Work out the finished part from the listing and answer in its coordinate system (mm). Coordinates: 2 decimals unless noted, no trailing zeros. Order: outer loops, then holes, each group sorted by start corner. A loop starts at its lowest first (then second) coordinate and runs counter-clockwise, first axis right, second up. Notation, with made-up numbers: (85, 77.5) -> (135, 77.5) arc R23 cw to (135, 104.5) -> close; hole circle Ø4 at (-30.5, 4.25). An arc over 180 degrees is marked (long way). Use one line per item in the form item = value.
from build123d import *

# Parameters (mm, degrees)
SKETCH_W     = 43.2
SKETCH_H     = 10.2
PAD_DEPTH    = 25.4
SKETCH001_R  = 0.55
PAD001_DEPTH = 5.97
SKETCH002_R  = 1.5
POCKET_DEPTH = 25.401


with BuildPart() as part:
    # Sketch → Pad (new body)
    with BuildSketch(Plane.XY):
        Rectangle(SKETCH_W, SKETCH_H)
    extrude(amount=PAD_DEPTH)

    # Sketch001 (on Face5 of Pad) → Pad001 (join)
    with BuildSketch(Plane(origin=(0, 0, 0), x_dir=(1, 0, 0), z_dir=(0, 0, -1))):
        with Locations((14, 2.6)):
            Circle(SKETCH001_R)
        with Locations((3.8, 2.6)):
            Circle(SKETCH001_R)
        with Locations((-8.9, 2.6)):
            Circle(SKETCH001_R)
        with Locations((-14, 2.6)):
            Circle(SKETCH001_R)
        with Locations((-19, 2.6)):
            Circle(SKETCH001_R)
    extrude(amount=PAD001_DEPTH)

    # Sketch002 (on Face4 of Pad001) → Pocket (cut, through all)
    with BuildSketch(Plane(origin=(0, 0, 0), x_dir=(1, 0, 0), z_dir=(0, 0, -1))):
        with Locations((-3.8, -2.5)):
            Circle(SKETCH002_R)
    extrude(amount=-POCKET_DEPTH, mode=Mode.SUBTRACT)


solid = part.part
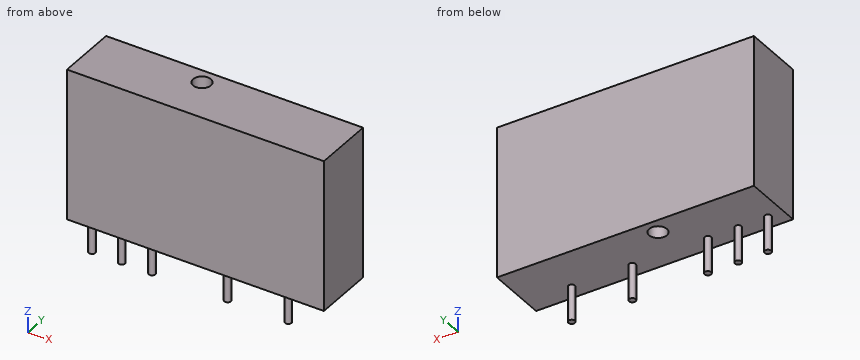
(1) Section B-B on y = 2.5 is taken. Write down the section's boundary in (x, z), plus the area to 3 significant figures.
Data:
outline = (-21.6, 0) -> (-5.3, 0) -> (-5.3, 25.4) -> (-21.6, 25.4) -> close; (-2.3, 0) -> (21.6, 0) -> (21.6, 25.4) -> (-2.3, 25.4) -> close
area = 1,020 mm²
(2) Straight lines are drawn through the part: line 1 along Y through (x, z) = (-3.8, 19.75); line 2 along X through (y, z) = (2.5, 17); line 3 along Z through (x, y) = (0, 0). For each, find the intervals that lie inside material, in ascending order.
Data:
line_1 = -5.1 to 1, 4 to 5.1
line_2 = -21.6 to -5.3, -2.3 to 21.6
line_3 = 0 to 25.4
(3) Section A-A on x = -3.8 is taken. Write down the section's boundary in (y, z).
Data:
outline = (-5.1, 0) -> (1, 0) -> (1, 25.4) -> (-5.1, 25.4) -> close; (4, 0) -> (5.1, 0) -> (5.1, 25.4) -> (4, 25.4) -> close
(4) Section D-D on y = -2.6 is taken. Write down the section's boundary in (x, z), plus the area to 3 significant figures.
Data:
outline = (-21.6, 0) -> (-19.55, 0) -> (-19.55, -5.97) -> (-18.45, -5.97) -> (-18.45, 0) -> (-14.55, 0) -> (-14.55, -5.97) -> (-13.45, -5.97) -> (-13.45, 0) -> (-9.45, 0) -> (-9.45, -5.97) -> (-8.35, -5.97) -> (-8.35, 0) -> (3.25, 0) -> (3.25, -5.97) -> (4.35, -5.97) -> (4.35, 0) -> (13.45, 0) -> (13.45, -5.97) -> (14.55, -5.97) -> (14.55, 0) -> (21.6, 0) -> (21.6, 25.4) -> (-21.6, 25.4) -> close
area = 1,130 mm²
(5) Section C-C on z = 15 is taken. Write down the section's boundary in (x, y).
Data:
outline = (-21.6, -5.1) -> (21.6, -5.1) -> (21.6, 5.1) -> (-21.6, 5.1) -> close; hole circle Ø3 at (-3.8, 2.5)
(6) This flat-tipped pin is pushed along its axis until it touches: P1, Ø5, axis at x = 14.5, y = 3.5, coming from the -Z side. Where does it stop, or does it pass through?
Data:
P1 = 0
